Verification items for the finished model (mm, model axes). Face numbers are marked on the shaded views. A direction names the side the tool comes from. Give positions to 0.01 mm unless a question says otherwise; leave off trailing zeros. Order: outer loops, then holes, each group sorted by start corner. A loop starts at its lowest first (then second) coordinate and runs counter-clockwise, first axis right, second up. Notation, with made-up numbers: (53, 40.5) - (79, 40.5) arc R32 ccw to (79, 69.5) - close; hole circle Ø6 at (33, 45). An arc over 180 degrees is marked (long way). Answer as a JSON object with one key per item and string values. Group by question number.
(1) Thickness scan on line 1 (Z direction, x = -1, y = 4.25); line 2 (Y direction, x = 0, z = 9); line 3 (X direction, y = 4.5, z = 2.25). Record the ranges inside material, lowest first.
(2) Access from +Z, -Z, +X, -X, +Y, -Y to the whole of each face (thin tool, end or side, straight path). Record for the marked faces 1 and 2.
(3) Depth check by flat-ended pin: pin 1 Ø4 at (y, z) = (-3, 8.5) entering from -X. Enter the tip coordinate at first touch or a pass-through.
(4) Section check C-C (z = 21.25). Record the boundary of the cut face in (x, y), then the cut area to 3 significant figures.
(5) Section check B-B (z = 2.25). Record the boundary of the cut face in (x, y), then the cut area to 3 significant figures.
```python
from build123d import *

# Parameters (mm, degrees)
Y_KSEKLIK_EKSTR_ZYON1_DEPTH = 4
IZIM3_R                     = 3
Y_KSEKLIK_EKSTR_ZYON2_DEPTH = 20
RADYUS1_R                   = 0.5


with BuildPart() as part:
    # Çizim1 → Yükseklik-Ekstrüzyon1 (new body)
    with BuildSketch(Plane.XY):
        Polygon((5.773502692, 0), (2.886751346, 5), (-2.886751346, 5), (-5.773502692, 0), (-2.886751346, -5), (2.886751346, -5), align=None)
    extrude(amount=Y_KSEKLIK_EKSTR_ZYON1_DEPTH)

    # Çizim2 → Kes-Döndür1 (revolve, cut)
    with BuildSketch(Plane(origin=(0, 0, 0), x_dir=(1, 0, 0), z_dir=(0, 1, 0))):
        Polygon((-5.773502692, 0), (-5.773502692, -0.5), (-4.973502692, 0), align=None)
        Polygon((-5.773502692, -4), (-5.773502692, -3.5), (-4.973502692, -4), align=None)
    revolve(axis=Axis((0, 0, 0), (0, 0, 1)), mode=Mode.SUBTRACT)

    # Çizim3 → Yükseklik-Ekstrüzyon2 (add)
    with BuildSketch(Plane.XY.offset(4)):
        Circle(IZIM3_R)
    extrude(amount=Y_KSEKLIK_EKSTR_ZYON2_DEPTH)

    # Radyus1
    radyus1_edges = [part.edges().sort_by_distance(p)[0] for p in [
        (-3, 0, 24),
    ]]
    fillet(radyus1_edges, radius=RADYUS1_R)


solid = part.part
```
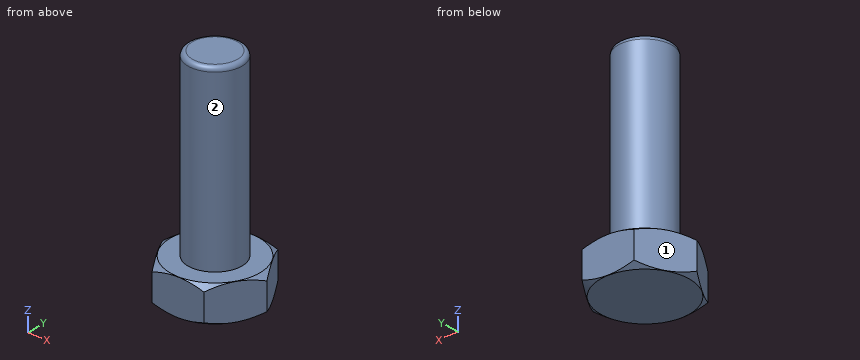
Solutions:
{
 "1": {"line 1": "z = 0 to 4", "line 2": "y = -3 to 3", "line 3": "x = -3.18 to 3.18"},
 "2": {"face 1": "+Z, -Z, -X, +Y", "face 2": "+Z"},
 "3": {"pin 1": "stops at x = -2.83"},
 "4": {"outline": "circle Ø6 at (0, 0)", "area": "28.3 mm2"},
 "5": {"outline": "(-5.77, 0) - (-2.89, -5) - (2.89, -5) - (5.77, 0) - (2.89, 5) - (-2.89, 5) - close", "area": "86.6 mm2"}
}
